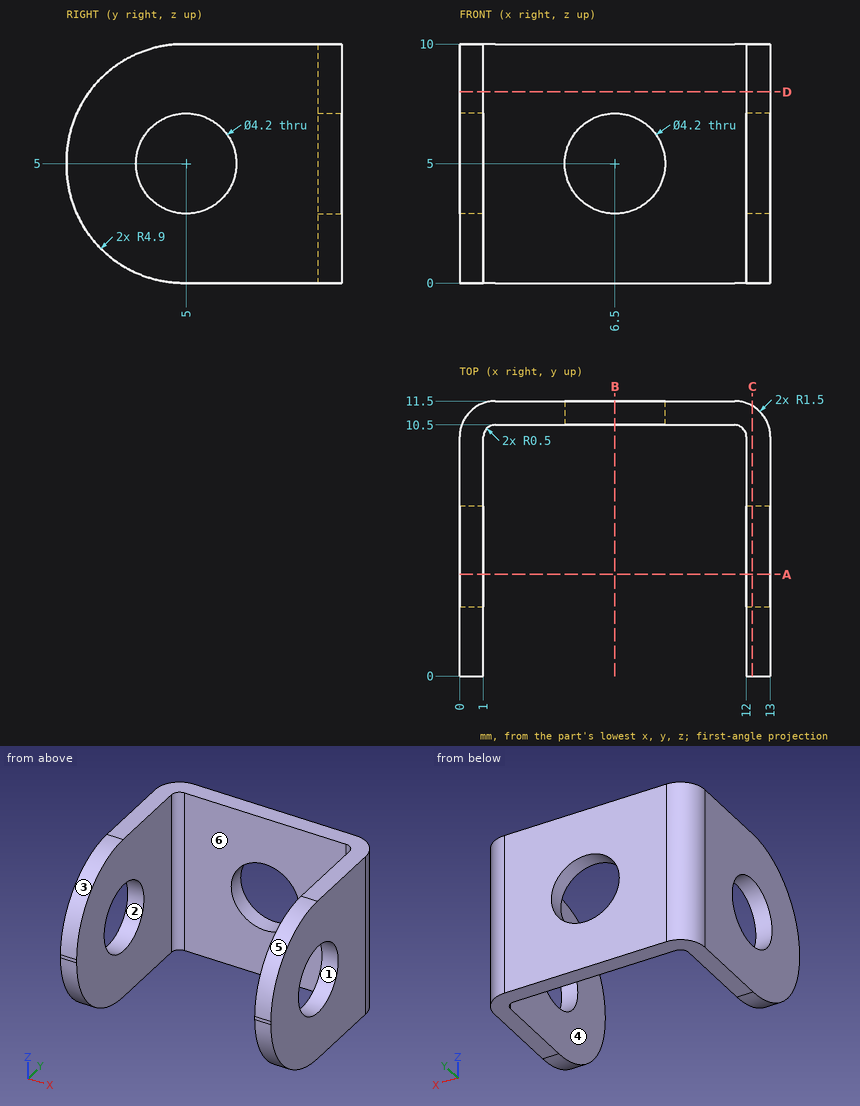
Verification items for this drawing (mm, ordinates from the low corner). A direction names the side the tool comes from. Round coordinates to 2 decimals unless told otherwise and drop trailing zeros. Loops run counter-clockwise (first coordinate to the right, second up) from the corner with the lowest first, then second, coordinate; pieces in that order, holes last. Notation, with made-up numbers: M 42,54.5 L 93,54.5 A15 ccw 93,64.5 Z; hole C -10.75,-39 d4. An arc over 180 degrees is marked long. Answer as a JSON object with one key per item and string values.
1. Section check B-B (x = 6.5). Record the boundary of the cut face in (y, z), plus the area to 3 significant figures.
Reply:
{"outline": "M 10.5,0 L 11.5,0 L 11.5,2.9 L 10.5,2.9 Z; M 10.5,7.1 L 11.5,7.1 L 11.5,10 L 10.5,10 Z", "area": "5.80 mm²"}
2. Section check A-A (y = 4.25). Record the boundary of the cut face in (x, z), plus the area to 3 significant figures.
Reply:
{"outline": "M 0,0.04 L 1,0.04 L 1,3.04 L 0,3.04 Z; M 0,6.96 L 1,6.96 L 1,9.96 L 0,9.96 Z; M 12,0.04 L 13,0.04 L 13,3.04 L 12,3.04 Z; M 12,6.96 L 13,6.96 L 13,9.96 L 12,9.96 Z", "area": "12.0 mm²"}
3. Gauge pin test, flat end, axial feed: P1, Ø1.5, axis at x = 8.5, y = 8, coming from the -Z side. Record the tip position at first contact, or that the pin passes through.
Reply:
{"P1": "passes through"}
4. Section check D-D (z = 8). Record the boundary of the cut face in (x, y), plus the area to 3 significant figures.
Reply:
{"outline": "M 0,0.95 L 1,0.95 L 1,10 A0.5 cw 1.5,10.5 L 11.5,10.5 A0.5 cw 12,10 L 12,0.95 L 13,0.95 L 13,10 A1.5 ccw 11.5,11.5 L 1.5,11.5 A1.5 ccw 0,10 Z", "area": "31.2 mm²"}
5. Section check C-C (x = 12.25). Record the boundary of the cut face in (y, z).
Reply:
{"outline": "M 0,4.9 A4.9 ccw 4.9,0 L 11.3,0 L 11.3,10 L 4.9,10 A4.9 ccw 0,5.1 Z; hole C 5,5 d4.2"}
6. Access from +Z, -Z, +X, -X, +Y, -Y to the whole of each face (thin tool, end or side, straight path). Record for the marked faces 5 and 6.
Reply:
{"face 5": "+Z, +X, -X, -Y", "face 6": "+Z, -Z, -Y"}
7. Scan lines: line 1 (Z direction, x = 0.5, y = 5); line 2 (X direction, y = 3.5, z = 7); line 3 (Y direction, x = 2.5, z = 4). Record each from-to range of solid material in increasing order.
Reply:
{"line 1": "z = 0 to 2.9, 7.1 to 10", "line 2": "x = 0 to 1, 12 to 13", "line 3": "y = 10.5 to 11.5"}
8. Mould release check, pull along Y, two halves, no side actions. Record for the marked faces 1, 2, 3 and 4: pulls with the +Y half, pulls with the -Y half, needs draft (parallel to the pull), parting line crosses it, or undercut.
Reply:
{"face 1": "undercut", "face 2": "undercut", "face 3": "pulls with the -Y half", "face 4": "needs draft"}
